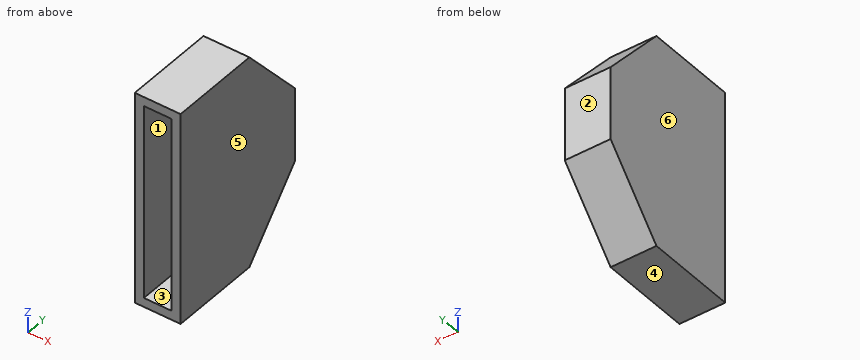
from build123d import *
from OCP.BRepFilletAPI import BRepFilletAPI_MakeChamfer

# Parameters (mm, degrees)
ESQUISSE1_W             = 15
ESQUISSE1_H             = 70
BOSS_EXTRU_1_DEPTH      = 50
CHANFREIN1_SIZE         = 20
CHANFREIN1_SIZE2        = 23.007368144
ESQUISSE2_W             = 9
ESQUISSE2_H             = 64
ENL_V_MAT_EXTRU_1_DEPTH = 30


with BuildPart() as part:
    # Esquisse1 → Boss.-Extru.1 (new body)
    with BuildSketch(Plane(origin=(0, 0, 0), x_dir=(1, 0, 0), z_dir=(0, 1, 0))):
        Rectangle(ESQUISSE1_W, ESQUISSE1_H)
    extrude(amount=BOSS_EXTRU_1_DEPTH)

    # Chanfrein1: one chamfer whose edges measure the first distance from different faces: ONE call of the kernel's chamfer builder (chamfer() names one face for all edges)
    chanfrein1_edges_1 = [part.edges().sort_by_distance(p)[0] for p in [
        (0, 50, -35),
    ]]
    chanfrein1_side_1 = [part.faces().sort_by_distance(p)[0] for p in [
        (0, 25, -35),
    ]]
    chanfrein1_edges_2 = [part.edges().sort_by_distance(p)[0] for p in [
        (0, 50, 35),
    ]]
    chanfrein1_side_2 = [part.faces().sort_by_distance(p)[0] for p in [
        (0, 25, 35),
    ]]
    chanfrein1 = BRepFilletAPI_MakeChamfer(part.part.solid().wrapped)
    for e in chanfrein1_edges_1:
        chanfrein1.Add(CHANFREIN1_SIZE, CHANFREIN1_SIZE2, e.wrapped, chanfrein1_side_1[0].wrapped)  # the first distance lies on this face
    for e in chanfrein1_edges_2:
        chanfrein1.Add(CHANFREIN1_SIZE, CHANFREIN1_SIZE2, e.wrapped, chanfrein1_side_2[0].wrapped)  # the first distance lies on this face
    add(Compound.cast(chanfrein1.Shape()), mode=Mode.REPLACE)

    # Esquisse2 → Enlèv. mat.-Extru.1 (cut)
    with BuildSketch(Plane.XZ):
        Rectangle(ESQUISSE2_W, ESQUISSE2_H)
    extrude(amount=-ENL_V_MAT_EXTRU_1_DEPTH, mode=Mode.SUBTRACT)


solid = part.part
Source: CAD feature listing. Evaluate the final solid. Frame: model axes, mm. Face numbers are marked on the shaded views. A direction names the side the tool comes from. Coordinates: 2 decimals unless noted, no trailing zeros. Loops run counter-clockwise (first coordinate to the right, second up) from the corner with the lowest first, then second, coordinate; pieces in that order, holes last. Notation, with made-up numbers: (-8, -14) - (14, -14) arc R24 cw to (14, 23) - close; hole circle Ø11 at (67, 59.25). An arc over 180 degrees is marked (long way). One line per item, written item: value. Start each with the question number.
1. Set-up query: the marked faces 1 and 2. Return all of +Z, -Z, +X, -X, +Y, -Y with unobstructed straight access to the full face (end or side cutting, diameter ignored); none if empty.
2. Section D-D (x = 0.5). Return the cut outline in (y, z), and give its area (3 significant figures).
3. Ray query, L1, parallel to X at y = 17, z = 1; L2, parallel to Z at x = 2.75, y = 14; L3, parallel to Y at x = -1, z = 5.5. Return the intervals inside material, ascending.
4. Mould query, pull axis X, two halves, no side actions, for the marked faces 3, 4, 5 and 6. Classes: pulls with the +X half, pulls with the -X half, needs draft (parallel to the pull), parting line crosses it, or undercut.
5. Section A-A (y = 18). Return the cut outline in (x, z).
6. Section C-C (z = 14). Return the cut outline in (x, y).
7. Contact query for flat-ended pins moving along their axis: P1, Ø1.5, axis at x = 5.5, z = -12, coming from the -Y side; P2, Ø2, axis at x = -3, y = 37.5, coming from the +Z side; P3, Ø3, axis at x = -3, z = 24.5, coming from the +Y side. Output: stop coordinate, or through.
8. Section B-B (x = -5.5). Return the cut outline in (y, z), and give its area (3 significant figures).
Verdict:
1. face 1: -Y
1. face 2: +Z, -Z, +X, -X, +Y
2. outline: (0, -35) - (30, -35) - (50, -11.99) - (50, 11.99) - (30, 35) - (0, 35) - (0, 32) - (30, 32) - (30, -32) - (0, -32) - close
2. area: 1,120 mm2
3. L1: x = -7.5 to -4.5, 4.5 to 7.5
3. L2: z = -35 to -32, 32 to 35
3. L3: y = 30 to 50
4. face 3: undercut
4. face 4: needs draft
4. face 5: pulls with the +X half
4. face 6: pulls with the -X half
5. outline: (-7.5, -35) - (7.5, -35) - (7.5, 35) - (-7.5, 35) - close; hole (-4.5, -32) - (4.5, -32) - (4.5, 32) - (-4.5, 32) - close
6. outline: (-7.5, 0) - (-4.5, 0) - (-4.5, 30) - (4.5, 30) - (4.5, 0) - (7.5, 0) - (7.5, 48.26) - (-7.5, 48.26) - close
7. P1: stops at y = 0
7. P2: stops at z = 27.52
7. P3: stops at y = 40.43
8. outline: (0, -35) - (30, -35) - (50, -11.99) - (50, 11.99) - (30, 35) - (0, 35) - close
8. area: 3,040 mm2
